Geometry check sheet. Reference: the model listing, model coordinates, mm. A direction names the side the tool comes from. Give positions to 0.01 mm unless a question says otherwise; leave off trailing zeros. Write each loop counter-clockwise with the first axis right and the second up, starting at its lowest first coordinate (ties: lowest second). Pieces come first, ordered by that corner, then holes. Notation, with made-up numbers: (38, 66) -> (44, 66) arc R8 ccw to (44, 71) -> close; hole circle Ø4 at (-12, -10). An arc over 180 degrees is marked (long way). Write item = value, one per line. Start each with the question number.
1. Mould release check, pull along X, two halves, no side actions. Record for faces 1 (the flat face through (-41, -9, 1)), 2 (the flat face through (-47, -13, 3)), 3 (the flat face through (-42.569, -12.536, 2.24)), 4 (the flat face through (-44, -9, 1.5)): pulls with the +X half, pulls with the -X half, needs draft (parallel to the pull), parting line crosses it, or undercut.
2. Set-up check for faces 5 (the flat face through (-47.5, -9, 1)), 6 (the flat face through (-45.947, -12.564, 2.24)), 7 (the flat face through (-42, -7.025, 2)): record each of +Z, -Z, +X, -X, +Y, -Y from which the full face is reachable in a straight line by a thin tool's end or side.
3. Cross-section at C-C, the plane y = -13.25. Record the cut outline in (x, z), plus the area to 3 significant figures.
4. Cross-section at B-B, the plane x = -44.25. Record the cut outline in (y, z) (3 decimals).
5. Depth check by flat-ended pin: P1, Ø3, axis at x = -44.25, y = -13.525, coming from the +Z side. Enter the tip coordinate at first touch or a pass-through.
6. Thickness scan on line 1 along Y through (x, z) = (-46.25, 2.3) (3 decimals); line 2 along Y through (x, z) = (-44.25, 0.4) (3 decimals); line 3 along X through (y, z) = (-13.5, 1.05). Record the ranges inside material, lowest first.
7. Cross-section at A-A, the plane z = 2.55. Record the cut outline in (x, y) (3 decimals).
8. Cross-section at D-D, the plane x = -46.75. Record the cut outline in (y, z) (3 decimals), plus the area to 4 significant figures.
```python
from build123d import *

# Parameters (mm, degrees)
SKETCH1_W           = 6.5
SKETCH1_H           = 4
SKETCH1_R           = 1.25
SKETCH1_H_2         = 4.5
BOSS_EXTRUDE1_DEPTH = 1.5
BOSS_EXTRUDE2_DEPTH = 1.5


with BuildPart() as part:
    # Sketch1 → Boss-Extrude1 (new body)
    # profile 1 of 3: a face of its own
    with BuildSketch(Plane.XY):
        with Locations((-44.25, -13.525)):
            Rectangle(SKETCH1_W, SKETCH1_H)
        with Locations((-44.25, -13.525)):
            Circle(SKETCH1_R, mode=Mode.SUBTRACT)
    # profile 2 of 3: a face of its own
    with BuildSketch(Plane.XY):
        with Locations((-44.25, -5.025)):
            Rectangle(SKETCH1_W, SKETCH1_H)
        with Locations((-44.25, -5.025)):
            Circle(SKETCH1_R, mode=Mode.SUBTRACT)
    # profile 3 of 3: a face of its own
    with BuildSketch(Plane.XY):
        with Locations((-44.25, -9.275)):
            Rectangle(SKETCH1_W, SKETCH1_H_2)
    extrude(amount=BOSS_EXTRUDE1_DEPTH)

    # Sketch2 → Boss-Extrude2 (add)
    with BuildSketch(Plane.XY.offset(1.5)):
        Polygon((-47.5, -3.025), (-47.5, -7.025), (-45.375833025, -7.025), (-45.375833025, -6.975), (-46.50166605, -5.025), (-45.375833025, -3.075), (-45.375833025, -3.025), align=None)
        Polygon((-43.124166975, -7.025), (-41, -7.025), (-41, -3.025), (-43.124166975, -3.025), (-43.124166975, -3.075), (-41.99833395, -5.025), (-43.124166975, -6.975), align=None)
        Polygon((-45.375833025, -11.575), (-45.375833025, -11.525), (-47.5, -11.525), (-47.5, -15.525), (-45.375833025, -15.525), (-45.375833025, -15.475), (-46.50166605, -13.525), align=None)
        Polygon((-41, -11.525), (-43.124166975, -11.525), (-43.124166975, -11.575), (-41.99833395, -13.525), (-43.124166975, -15.475), (-43.124166975, -15.525), (-41, -15.525), align=None)
    extrude(amount=BOSS_EXTRUDE2_DEPTH)


solid = part.part
```
Answers:
q1.face_1 = pulls with the +X half
q1.face_2 = needs draft
q1.face_3 = undercut
q1.face_4 = undercut
q2.face_5 = +Z, -Z, -X, +Y, -Y
q2.face_6 = +Z
q2.face_7 = +Z, +X, -X
q3.outline = (-47.5, 0) -> (-45.47, 0) -> (-45.47, 1.5) -> (-46.34, 1.5) -> (-46.34, 3) -> (-47.5, 3) -> close; (-43.03, 0) -> (-41, 0) -> (-41, 3) -> (-42.16, 3) -> (-42.16, 1.5) -> (-43.03, 1.5) -> close
q3.area = 9.56 mm^2
q4.outline = (-15.525, 0) -> (-14.775, 0) -> (-14.775, 1.5) -> (-15.525, 1.5) -> close; (-12.275, 0) -> (-6.275, 0) -> (-6.275, 1.5) -> (-12.275, 1.5) -> close; (-3.775, 0) -> (-3.025, 0) -> (-3.025, 1.5) -> (-3.775, 1.5) -> close
q5.P1 = 1.5
q6.line_1 = -15.525 to -13.961, -13.089 to -11.525, -7.025 to -5.461, -4.589 to -3.025
q6.line_2 = -15.525 to -14.775, -12.275 to -6.275, -3.775 to -3.025
q6.line_3 = -47.5 to -45.5, -43 to -41
q7.outline = (-47.5, -15.525) -> (-45.376, -15.525) -> (-45.376, -15.475) -> (-46.502, -13.525) -> (-45.376, -11.575) -> (-45.376, -11.525) -> (-47.5, -11.525) -> close; (-47.5, -7.025) -> (-45.376, -7.025) -> (-45.376, -6.975) -> (-46.502, -5.025) -> (-45.376, -3.075) -> (-45.376, -3.025) -> (-47.5, -3.025) -> close; (-43.124, -15.525) -> (-41, -15.525) -> (-41, -11.525) -> (-43.124, -11.525) -> (-43.124, -11.575) -> (-41.998, -13.525) -> (-43.124, -15.475) -> close; (-43.124, -7.025) -> (-41, -7.025) -> (-41, -3.025) -> (-43.124, -3.025) -> (-43.124, -3.075) -> (-41.998, -5.025) -> (-43.124, -6.975) -> close
q8.outline = (-15.525, 0) -> (-3.025, 0) -> (-3.025, 3) -> (-7.025, 3) -> (-7.025, 1.5) -> (-11.525, 1.5) -> (-11.525, 3) -> (-15.525, 3) -> close
q8.area = 30.75 mm^2
